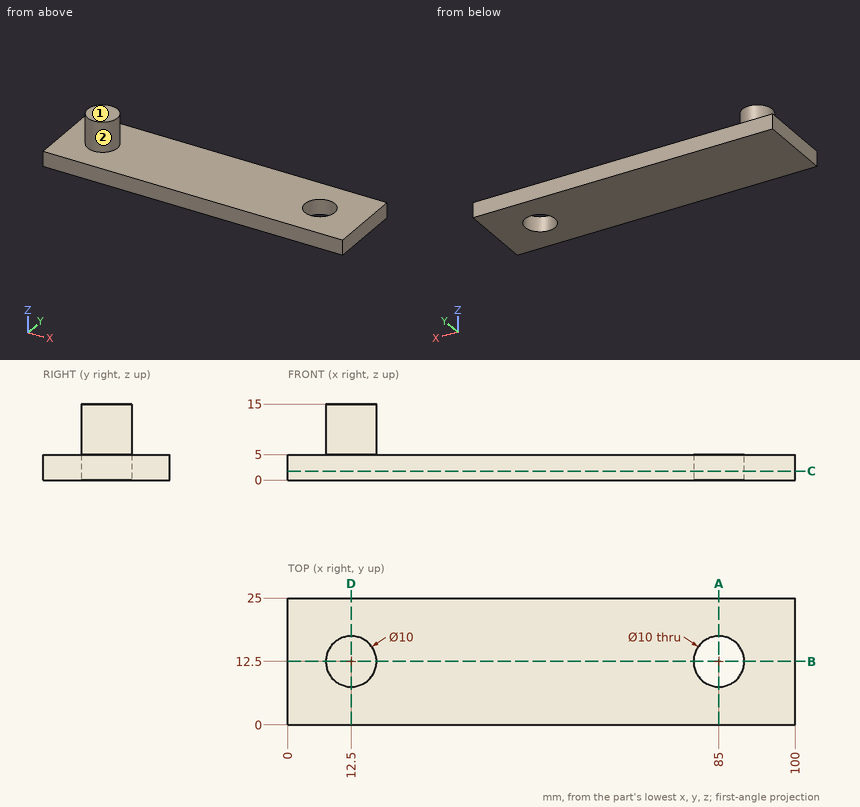
The figure shows three views and two pictorial views of one solid part (mm, origin at its lowest corner). Answer the questions. A direction names the side the tool comes from. Coordinates: 2 decimals unless noted, no trailing zeros. Order: outer loops, then holes, each group sorted by start corner. A loop starts at its lowest first (then second) coordinate and runs counter-clockwise, first axis right, second up. Notation, with made-up numbers: M -15.5,33.5 L 41.5,33.5 A9 cw 41.5,41.5 Z; hole C 1.5,87 d11. An arc over 180 degrees is marked long. Use CSV: the item, a comma, the result in double quotes.
1) Flat-ended cylindrical pins translate along their axes: pin 1 Ø12.5 at (x, y) = (56.5, 9.5) entering from +Z; pin 2 Ø2 at (y, z) = (8, 2.5) entering from -X; pin 3 Ø8 at (x, z) = (21, 10) entering from -Y. Find the tip coordinate at first contact, or state that the pin passes through.
Worked out:
pin 1,"stops at z = 5"
pin 2,"stops at x = 0"
pin 3,"stops at y = 10.32"
2) For the marked faces 1 and 2, determine the directions among +Z, -Z, +X, -X, +Y, -Y from which every point of the face is accessible in a straight line to the end or side of a thin tool.
Worked out:
face 1,"+Z, +X, -X, +Y, -Y"
face 2,"+Z"
3) Consider line 1 (Y direction, x = 85, z = 3.95); line 2 (Z direction, x = 63.5, y = 21.75); line 3 (X direction, y = 8.25, z = 13.5). Determine where each line is inside the solid, lowest interval first. Write a range as [from, to].
Worked out:
line 1,"y = [0, 7.5], [17.5, 25]"
line 2,"z = [0, 5]"
line 3,"x = [9.87, 15.13]"
4) Section C-C on z = 1.75 is taken. Write down the section's boundary in (x, y).
Worked out:
outline,"M 0,0 L 100,0 L 100,25 L 0,25 Z; hole C 85,12.5 d10"
5) Section A-A on x = 85 is taken. Write down the section's boundary in (y, z).
Worked out:
outline,"M 0,0 L 7.5,0 L 7.5,5 L 0,5 Z; M 17.5,0 L 25,0 L 25,5 L 17.5,5 Z"
6) Section B-B on y = 12.5 is taken. Write down the section's boundary in (x, z), plus the area to 3 significant figures.
Worked out:
outline,"M 0,0 L 80,0 L 80,5 L 17.5,5 L 17.5,15 L 7.5,15 L 7.5,5 L 0,5 Z; M 90,0 L 100,0 L 100,5 L 90,5 Z"
area,"550 mm^2"
7) Section D-D on x = 12.5 is taken. Write down the section's boundary in (y, z).
Worked out:
outline,"M 0,0 L 25,0 L 25,5 L 17.5,5 L 17.5,15 L 7.5,15 L 7.5,5 L 0,5 Z"
